from build123d import *

# Parameters (mm, degrees)
BOSS_EXTRUDE1_DEPTH = 65
FILLET1_R           = 13
SKETCH3_W           = 90
SKETCH3_H           = 70
CUT_EXTRUDE1_DEPTH  = 52


with BuildPart() as part:
    # Sketch2 → Boss-Extrude1 (new body)
    with BuildSketch(Plane(origin=(0, 0, 0), x_dir=(0, 0, -1), z_dir=(1, 0, 0))):
        Polygon((0, 0), (0, 85), (50, 85), (65, 100), (215, 100), (230, 85), (320, 85), (350, 55), (350, 0), (230, 0), (225, 5), (125, 5), (120, 0), align=None)
    extrude(amount=BOSS_EXTRUDE1_DEPTH)

    # Fillet1
    fillet1_edges = [part.edges().sort_by_distance(p)[0] for p in [
        (32.5, 0, 0),
        (32.5, 85, 0),
    ]]
    fillet(fillet1_edges, radius=FILLET1_R)

    # Sketch3 → Cut-Extrude1 (cut)
    with BuildSketch(Plane(origin=(65, 0, 0), x_dir=(0, 0, -1), z_dir=(1, 0, 0))):
        with Locations((58, 35)):
            Rectangle(SKETCH3_W, SKETCH3_H)
        with Locations((280, 35)):
            Rectangle(SKETCH3_W, SKETCH3_H)
    extrude(amount=-CUT_EXTRUDE1_DEPTH, mode=Mode.SUBTRACT)


solid = part.part
Design review of the part built by this model. Coordinates are the model's own, in mm. A direction names the side the tool comes from. Coordinates: 2 decimals unless noted, no trailing zeros. Loops run counter-clockwise (first coordinate to the right, second up) from the corner with the lowest first, then second, coordinate; pieces in that order, holes last. Notation, with made-up numbers: M 34.25,75.25 L 75.25,75.25 A24 ccw 75.25,112.25 Z; hole C 66,-14.5 d5. An arc over 180 degrees is marked long. Answer as CSV lines item,"result".
Item 1: For probe 1 along Z at (x, y) = (14, 21.5); probe 2 along Z at (x, y) = (37, 56); probe 3 along Y at (x, z) = (53, -307), list the stretches that pass through material, from the lowest coordinate up.
Answer list:
probe 1,"-350 to -325, -235 to -103, -13 to 0"
probe 2,"-349 to -325, -235 to -103, -13 to 0"
probe 3,"70 to 85"
Item 2: Add section D-D on x = 5. State the section outline as (y, z) points, plus the area to 3 significant figures.
Answer list:
outline,"M 0,-350 L 55,-350 L 85,-320 L 85,-230 L 100,-215 L 100,-65 L 85,-50 L 85,-13 A13 ccw 72,0 L 13,0 A13 ccw 0,-13 L 0,-120 L 5,-125 L 5,-225 L 0,-230 Z"
area,"31,200 mm²"
Item 3: The part is to be moulded in two halves that separate along Z. For faces 1 (the face through (39, 35, -325)), 2 (the face through (32, 92, -57)), 3 (the face through (65, 62, -177)), say which applies: pulls with the +Z half, pulls with the -Z half, needs draft (parallel to the pull), parting line crosses it, or undercut.
Answer list:
face 1,"undercut"
face 2,"pulls with the +Z half"
face 3,"needs draft"
Item 4: Add section B-B on z = -291. State the section outline as (x, y) points.
Answer list:
outline,"M 0,0 L 13,0 L 13,70 L 65,70 L 65,85 L 0,85 Z"
Item 5: For P1, Ø12, axis at y = 32.5, z = -280, coming from the +X side; P2, Ø6, axis at x = 16, y = 76, coming from the +Z side, all flat-tipped, find the tip position at first contact; note any pin that passes through.
Answer list:
P1,"x = 13"
P2,"z = -0.04"
Item 6: Add section A-A on y = 47. State the section outline as (x, z) points.
Answer list:
outline,"M 0,-350 L 65,-350 L 65,-325 L 13,-325 L 13,-235 L 65,-235 L 65,-103 L 13,-103 L 13,-13 L 65,-13 L 65,0 L 0,0 Z"
Item 7: Machinability: for faces 4 (the face through (13, 35, -57)), 5 (the face through (10, 0, -318)), 6 (the face through (32, 85, -31)), 7 (the face through (32, 85, -274)), 8 (the face through (32, 5, -176)), which of the approach directions +Z, -Z, +X, -X, +Y, -Y give a long, thin tool a straight path to every point of the face, cutting with its end or side? Answer none if there is none.
Answer list:
face 4,"+X, -Y"
face 5,"+Z, -Z, +X, -X, -Y"
face 6,"+Z, +X, -X, +Y"
face 7,"-Z, +X, -X, +Y"
face 8,"+X, -X, -Y"
Item 8: Add section C-C on x = 40. State the section outline as (y, z) points, plus the area to 3 significant figures.
Answer list:
outline,"M 0,-350 L 55,-350 L 85,-320 L 85,-230 L 100,-215 L 100,-65 L 85,-50 L 85,-13 A13 ccw 72,0 L 13,0 A13 ccw 0,-13 L 70,-13 L 70,-103 L 0,-103 L 0,-120 L 5,-125 L 5,-225 L 0,-230 L 0,-235 L 70,-235 L 70,-325 L 0,-325 Z"
area,"18,600 mm²"
